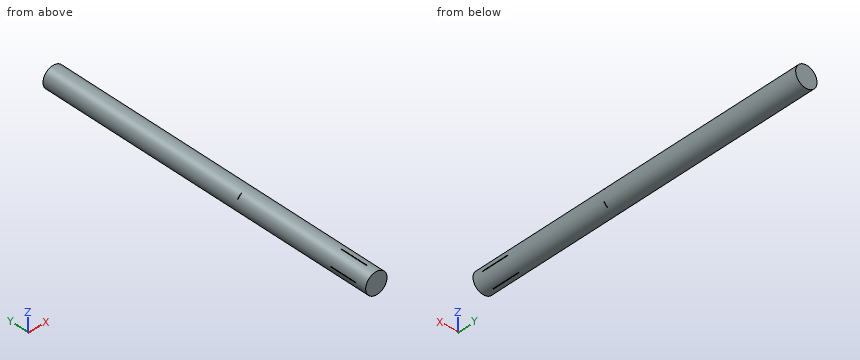
from build123d import *

# Parameters (mm, degrees)
SKETCH1_R           = 77.6224
SKETCH1_R_2         = 76.2
BOSS_EXTRUDE1_DEPTH = 2565.4
SKETCH2_W           = 4.7625
SKETCH2_H           = 203.2
CUT_EXTRUDE1_DEPTH  = 2568.747579877
CIRPATTERN1_COUNT   = 4
SKETCH3_W           = 38.1
SKETCH3_H           = 3.175
CUT_EXTRUDE2_DEPTH  = 2568.747579877
CIRPATTERN2_COUNT   = 4
SKETCH4_R           = 76.2
BOSS_EXTRUDE2_DEPTH = 2565.4


with BuildPart() as part:
    # Sketch1 → Boss-Extrude1 (new body)
    with BuildSketch(Plane(origin=(0, 0, 0), x_dir=(1, 0, 0), z_dir=(0, 1, 0))):
        with Locations(Location((0, 0, 0), (0, 0, 90))):
            Circle(SKETCH1_R)
        with Locations(Location((0, 0, 0), (0, 0, 90))):
            Circle(SKETCH1_R_2, mode=Mode.SUBTRACT)
    extrude(amount=BOSS_EXTRUDE1_DEPTH)

    # Sketch2 → Cut-Extrude1 (cut, through all)
    with BuildSketch(Plane.XY):
        with Locations((0, 177.8)):
            Rectangle(SKETCH2_W, SKETCH2_H)
    cut_extrude1 = extrude(amount=-CUT_EXTRUDE1_DEPTH, mode=Mode.SUBTRACT)

    # CirPattern1: Cut-Extrude1 ×4 about axis
    cirpattern1_axis = Axis((0, 0, 0), (0, 1, 0))
    for i in range(1, CIRPATTERN1_COUNT):
        add(cut_extrude1.rotate(cirpattern1_axis, i * 360 / CIRPATTERN1_COUNT), mode=Mode.SUBTRACT)

    # Sketch3 → Cut-Extrude2 (cut, through all)
    with BuildSketch(Plane(origin=(0, 0, 0), x_dir=(0.7071067811865477, 0, 0.7071067811865475), z_dir=(-0.7071067811865475, 0, 0.7071067811865477))):
        with Locations((0, 1029.0175)):
            Rectangle(SKETCH3_W, SKETCH3_H)
    cut_extrude2 = extrude(amount=-CUT_EXTRUDE2_DEPTH, mode=Mode.SUBTRACT)

    # CirPattern2: Cut-Extrude2 ×4 about axis
    cirpattern2_axis = Axis((0, 0, 0), (0, 1, 0))
    for i in range(1, CIRPATTERN2_COUNT):
        add(cut_extrude2.rotate(cirpattern2_axis, i * 360 / CIRPATTERN2_COUNT), mode=Mode.SUBTRACT)

    # Sketch4 → Boss-Extrude2 (add)
    with BuildSketch(Plane.XZ):
        Circle(SKETCH4_R)
    extrude(amount=-BOSS_EXTRUDE2_DEPTH)


solid = part.part
Source: CAD feature listing. Evaluate the final solid. Frame: model axes, mm. Coordinates: 2 decimals unless noted, no trailing zeros. Loops run counter-clockwise (first coordinate to the right, second up) from the corner with the lowest first, then second, coordinate; pieces in that order, holes last. Notation, with made-up numbers: M 80.25,89 L 132.25,89 A25 ccw 132.25,128 Z; hole C 79.25,36 d10. An arc over 180 degrees is marked long. Answer in a Markdown table with one row per item.
Q1. Ray query, probe 1 along Z at (x, y) = (5.5, 228.5); probe 2 along X at (y, z) = (287, 15.5); probe 3 along Z at (x, y) = (1, 1846.5). Return the intervals inside material, ascending. Write a range as from..to.
Answers below:
| item | result |
|---|---|
| probe 1 | z = -77.43..77.43 |
| probe 2 | x = -76.06..76.06 |
| probe 3 | z = -77.62..77.62 |
Q2. Section A-A on y = 208.5. Return the cut outline in (x, z), plus the area to 3 significant figures.
Answers below:
| item | result |
|---|---|
| outline | M -77.59,-2.38 A77.62 ccw -2.38,-77.59 L -2.38,-76.16 A76.2 ccw 2.38,-76.16 L 2.38,-77.59 A77.62 ccw 77.59,-2.38 L 76.16,-2.38 A76.2 ccw 76.16,2.38 L 77.59,2.38 A77.62 ccw 2.38,77.59 L 2.38,76.16 A76.2 ccw -2.38,76.16 L -2.38,77.59 A77.62 ccw -77.59,2.38 L -76.16,2.38 A76.2 ccw -76.16,-2.38 Z |
| area | 18,900 mm^2 |
Q3. First-contact query: pin 1 (10 mm diameter, centred on y = 616, z = 39.5, fed in from +X); pin 2 (1.5 mm diameter, centred on y = 518.5, z = 11.5, fed in from -X); pin 3 (6 mm diameter, centred on y = 1484, z = 18, fed in from -X); pin 4 (14 mm diameter, centred on x = 53.5, z = 48.5, fed in from -Y). Flat tips, straight axial feed; report the tip coordinate or a pass-through.
Answers below:
| item | result |
|---|---|
| pin 1 | stops at x = 69.53 |
| pin 2 | stops at x = -76.87 |
| pin 3 | stops at x = -76.16 |
| pin 4 | stops at y = 0 |
Q4. Section B-B on y = 2032.5. Return the cut outline in (x, z), plus the area to 3 significant figures.
Answers below:
| item | result |
|---|---|
| outline | C 0,0 d155.24 |
| area | 18,900 mm^2 |
